Verification items for the finished model (mm, model axes). Face numbers are marked on the shaded views. A direction names the side the tool comes from. Coordinates: 2 decimals unless noted, no trailing zeros. Write each loop counter-clockwise with the first axis right and the second up, starting at its lowest first coordinate (ties: lowest second). Pieces come first, ordered by that corner, then holes. Notation, with made-up numbers: (59.5, 89) -> (104.5, 89) arc R28 ccw to (104.5, 125) -> close; hole circle Ø1 at (10, 32). An arc over 180 degrees is marked (long way). Answer in a Markdown table with one row per item.
```python
from build123d import *

# Parameters (mm, degrees)
F0_R     = 5.5
F1_DEPTH = 10
F3_DEPTH = 137.8111356168
F4_REACH = 250.1802781517
F5_R     = 5
F6_DEPTH = 152.6664515987
F7_R     = 5
F8_DEPTH = 35.9817621135


with BuildPart() as f1:
    # F0 (on Top) → F1 (new body)
    with BuildSketch(Plane.XY):
        with BuildLine():
            ThreePointArc((-114.9011806829, 81.9265817605), (-131.2129171427, 73.936702076), (-137.8111356168, 57.0141007194))
            Line((-137.8111356168, 57.0141007194), (-137.8111356168, -32.9858992806))
            Line((-137.8111356168, -32.9858992806), (25.1888643832, -32.9858992806))
            Line((25.1888643832, -32.9858992806), (26.0714058339, 0.8295803985))
            ThreePointArc((26.0714058339, 0.8295803985), (30.9682705236, 15.0503307045), (43.1380721252, 23.8880313122))
            Line((43.1380721252, 23.8880313122), (130.3572190405, 53.0392771455))
            ThreePointArc((130.3572190405, 53.0392771455), (146.9184021007, 81.7933335256), (120.3423502221, 101.6624555296))
            Line((120.3423502221, 101.6624555296), (-114.9011806829, 81.9265817605))
        make_face()
        with Locations((-112.8111356168, -12.4858992806)):
            Circle(F0_R, mode=Mode.SUBTRACT)
        Circle(F0_R, mode=Mode.SUBTRACT)
        with Locations((-112.8111356168, 57.0141007194)):
            Circle(F0_R, mode=Mode.SUBTRACT)
        with Locations((122.4323952882, 76.7499744885)):
            Circle(F0_R, mode=Mode.SUBTRACT)
    extrude(amount=F1_DEPTH)

    # F2 (on Right) → F3 (join, through all)
    with BuildSketch(Plane.YZ):
        Polygon((-38.7594019725, 10), (-66.6461533184, -38.3012701892), (-109.9474235076, -13.3012701892), (-114.9474235076, -21.9615242271), (-62.9858992806, -51.9615242271), (-32.9858992806, 0), (-32.9858992806, 10), align=None)
    extrude(amount=-F3_DEPTH)

    f4_end = Plane(origin=(25.6301351085, -16.078159441, 5), x_dir=(0.0260898572, 0.9996596017, 0), z_dir=(0.9996596017, -0.0260898572, 0))
    # F2 (on Right) → F4 (join, up to a plane its end follows)
    with BuildSketch(Plane.YZ):
        Polygon((-38.7594019725, 10), (-66.6461533184, -38.3012701892), (-109.9474235076, -13.3012701892), (-114.9474235076, -21.9615242271), (-62.9858992806, -51.9615242271), (-32.9858992806, 0), (-32.9858992806, 10), align=None)
    f4_long = extrude(amount=F4_REACH, mode=Mode.PRIVATE)
    add(split(f4_long, bisect_by=f4_end, keep=Keep.BOTTOM, mode=Mode.PRIVATE))

    # F5 (on face) → F6 (cut, through all)
    with BuildSketch(Plane(origin=(0, -33.3996784983, 19.2833133718), x_dir=(1, 0, 0), z_dir=(0, -0.8660254038, 0.5))):
        with Locations((-84.6435874701, -42.7307449281)):
            Circle(F5_R)
        with Locations((-37.48293221, -42.7307449281)):
            Circle(F5_R)
    extrude(amount=-F6_DEPTH, mode=Mode.SUBTRACT)

    # F7 (on face) → F8 (cut, through all)
    with BuildSketch(Plane(origin=(0, -33.2464748201, -57.584583561), x_dir=(1, 0, 0), z_dir=(0, 0.5, 0.8660254038))):
        with Locations((-97.8111356168, -55.862698704)):
            Circle(F7_R)
        with Locations((-17.8111356168, -55.862698704)):
            Circle(F7_R)
    extrude(amount=-F8_DEPTH, mode=Mode.SUBTRACT)


solid = f1.part
```
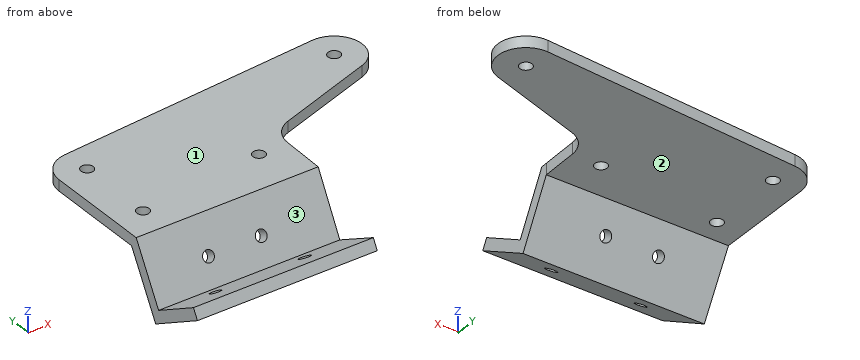
1. Tool access check on the marked faces 1, 2 and 3. Record the directions out of +Z, -Z, +X, -X, +Y, -Y that give a thin tool (end or side, any length) a straight path to the whole face; none if there is none.
Geometry says:
| item | result |
|---|---|
| face 1 | +Z, +X, -X, +Y, -Y |
| face 2 | -Z, +X, -X, +Y |
| face 3 | +Z, +X, -X |
2. Section check B-B, the plane x = 123.5. Record the boundary of the cut face in (y, z), plus the area to 3 significant figures.
Geometry says:
| item | result |
|---|---|
| outline | (50.75, 0) -> (71.35, 0) -> (71.35, 10) -> (50.75, 10) -> close; (82.15, 0) -> (101.73, 0) -> (101.73, 10) -> (82.15, 10) -> close |
| area | 402 mm^2 |
3. Section check C-C, the plane y = -21. Record the boundary of the cut face in (x, z).
Geometry says:
| item | result |
|---|---|
| outline | (-137.81, 0) -> (25.5, 0) -> (25.5, 10) -> (-137.81, 10) -> close |
4. Section check A-A, the plane x = -19. Record the boundary of the cut face in (y, z), plus the area to 3 significant figures.
Geometry says:
| item | result |
|---|---|
| outline | (-114.95, -21.96) -> (-90.83, -35.89) -> (-85.83, -27.22) -> (-109.95, -13.3) -> close; (-82.42, -40.74) -> (-62.99, -51.96) -> (-32.99, 0) -> (89.97, 0) -> (89.97, 10) -> (-38.76, 10) -> (-66.65, -38.3) -> (-77.42, -32.08) -> close |
| area | 2,290 mm^2 |
5. Thickness scan on line 1 (X direction, y = -79, z = -33); line 2 (Z direction, x = 96, y = 90); line 3 (Y direction, x = -43.5, z = -37.5). Record the ranges inside material, lowest first. Write a range as from..to.
Geometry says:
| item | result |
|---|---|
| line 1 | -137.81..-100.88, -94.74..-20.88, -14.74..23.99 |
| line 2 | 0..10 |
| line 3 | -88.03..-68.03, -66.18..-54.64 |
6. Section check D-D, the plane z = -7.5. Record the boundary of the cut face in (x, y).
Geometry says:
| item | result |
|---|---|
| outline | (-137.81, -48.86) -> (24.77, -48.86) -> (25.08, -37.32) -> (-137.81, -37.32) -> close |
7. Depth check by flat-ended pin: P1, Ø5, axis at x = -51.5, y = 57.5, coming from the -Z side; P2, Ø6, axis at y = -56.5, z = -40.5, coming from the +X side; P3, Ø8, axis at x = 16, z = -18, coming from the +Y side. Enter the tip coordinate at first touch or a pass-through.
Geometry says:
| item | result |
|---|---|
| P1 | z = 0 |
| P2 | x = 24.62 |
| P3 | y = -41.07 |
